Here's how the part is built. I have some questions about the finished solid (model axes, mm). Face numbers are marked on the shaded views. A direction names the side the tool comes from. Give positions to 0.01 mm unless a question says otherwise; leave off trailing zeros. Use one line per item in the form item = value. Start each with the question number.
from build123d import *

# Parameters (mm, degrees)
SKETCH2_R               = 3.127
SKETCH2_W               = 26.7
SKETCH2_H               = 32.3
BOSS_EXTRUDE1_DEPTH     = 10
CUT_EXTRUDE1_DEPTH      = 52.979378239
CUT_EXTRUDE1_DEPTH_BACK = 52.979378239
CUT_EXTRUDE2_DEPTH      = 52.979378239
CUT_EXTRUDE2_DEPTH_BACK = 52.979378239
CUT_EXTRUDE3_REACH      = 60.213
CUT_EXTRUDE3_END_RADIUS = 3.127
SKETCH6_W               = 4.772967813
SKETCH6_H               = 4
CUT_EXTRUDE4_REACH      = 60.213
CUT_EXTRUDE4_END_RADIUS = 3.127
SKETCH7_W               = 4.772967813
SKETCH7_H               = 4
CUT_EXTRUDE5_REACH      = 60.213
CUT_EXTRUDE5_END_RADIUS = 3.127
SKETCH8_W               = 4.772967813
SKETCH8_H               = 4
CUT_EXTRUDE6_REACH      = 60.213
CUT_EXTRUDE6_END_RADIUS = 3.127
SKETCH9_W               = 4.772967813
SKETCH9_H               = 4
SKETCH10_W              = 1.2
SKETCH10_H              = 12.610624374
SKETCH10_W_2            = 7.1
SKETCH10_H_2            = 1.2
SKETCH10_H_3            = 12.7
BOSS_EXTRUDE2_DEPTH     = 4
CUT_EXTRUDE7_DEPTH      = 3
CUT_EXTRUDE9_DEPTH      = 3
SKETCH13_W              = 7.833075365
SKETCH13_H              = 0.6
BOSS_EXTRUDE3_DEPTH     = 1.2
CHAMFER1_SIZE           = 1.2
SKETCH14_W              = 7.833075365
SKETCH14_H              = 0.6
BOSS_EXTRUDE4_DEPTH     = 1.2
CHAMFER2_SIZE           = 1.2


with BuildPart() as part:
    # Sketch2 → Boss-Extrude1 (new body)
    with BuildSketch(Plane(origin=(0, 0, 0), x_dir=(1, 0, 0), z_dir=(0, 1, 0))):
        with BuildLine():
            Line((-34.405486348, 30.435899661), (-24.03957695, 12.074655042))
            Line((-24.03957695, 12.074655042), (-24.03957695, -0.625344958))
            Line((-24.03957695, -0.625344958), (-34.405486348, -18.986589577))
            ThreePointArc((-34.405486348, -18.986589577), (-33.424886075, -24.740002888), (-27.671446386, -23.75955739))
            Line((-27.671446386, -23.75955739), (-13.03957695, -11.625344958))
            Line((-13.03957695, -11.625344958), (-5.93957695, -11.625344958))
            Line((-5.93957695, -11.625344958), (8.692292487, -23.75955739))
            ThreePointArc((8.692292487, -23.75955739), (14.445732176, -24.740002888), (15.426332449, -18.986589577))
            Line((15.426332449, -18.986589577), (5.06042305, -0.625344958))
            Line((5.06042305, -0.625344958), (5.06042305, 12.074655042))
            Line((5.06042305, 12.074655042), (15.426332449, 30.435899661))
            ThreePointArc((15.426332449, 30.435899661), (14.445732176, 36.189312973), (8.692292487, 35.208867474))
            Line((8.692292487, 35.208867474), (-5.93957695, 23.074655042))
            Line((-5.93957695, 23.074655042), (-13.03957695, 23.074655042))
            Line((-13.03957695, 23.074655042), (-27.671446386, 35.208867474))
            ThreePointArc((-27.671446386, 35.208867474), (-33.424886075, 36.189312973), (-34.405486348, 30.435899661))
        make_face()
        with Locations(Location((-31.038402168, 32.82229299, 0), (0, 0, 270))):
            Circle(SKETCH2_R, mode=Mode.SUBTRACT)
        with Locations(Location((12.059248268, 32.82229299, 0), (0, 0, 90))):
            Circle(SKETCH2_R, mode=Mode.SUBTRACT)
        with Locations(Location((-31.038402168, -21.372982906, 0), (0, 0, 90))):
            Circle(SKETCH2_R, mode=Mode.SUBTRACT)
        with Locations(Location((12.059248268, -21.372982906, 0), (0, 0, 270))):
            Circle(SKETCH2_R, mode=Mode.SUBTRACT)
        with BuildLine():
            Line((-24.03957695, 23.074655042), (-14.606114632, 23.074655042))
            Line((-14.606114632, 23.074655042), (-26.939458612, 33.302699824))
            ThreePointArc((-26.939458612, 33.302699824), (-28.459986314, 29.599886951), (-32.406136372, 28.928524617))
            Line((-32.406136372, 28.928524617), (-24.03957695, 14.108749692))
            Line((-24.03957695, 14.108749692), (-24.03957695, 23.074655042))
        make_face(mode=Mode.SUBTRACT)
        with Locations((-9.48957695, 5.724655042)):
            Rectangle(SKETCH2_W, SKETCH2_H, mode=Mode.SUBTRACT)
        with BuildLine():
            Line((5.06042305, 23.074655042), (5.06042305, 14.108749692))
            Line((5.06042305, 14.108749692), (13.426982473, 28.928524617))
            ThreePointArc((13.426982473, 28.928524617), (9.480832414, 29.599886951), (7.960304713, 33.302699824))
            Line((7.960304713, 33.302699824), (-4.373039267, 23.074655042))
            Line((-4.373039267, 23.074655042), (5.06042305, 23.074655042))
        make_face(mode=Mode.SUBTRACT)
        with BuildLine():
            Line((-24.03957695, -11.625344958), (-14.606114632, -11.625344958))
            Line((-14.606114632, -11.625344958), (-26.939458612, -21.85338974))
            ThreePointArc((-26.939458612, -21.85338974), (-28.459986314, -18.150576866), (-32.406136372, -17.479214533))
            Line((-32.406136372, -17.479214533), (-24.03957695, -2.659439608))
            Line((-24.03957695, -2.659439608), (-24.03957695, -11.625344958))
        make_face(mode=Mode.SUBTRACT)
        with BuildLine():
            Line((7.960304713, -21.85338974), (-4.373039267, -11.625344958))
            Line((-4.373039267, -11.625344958), (5.06042305, -11.625344958))
            Line((5.06042305, -11.625344958), (5.06042305, -2.659439608))
            Line((5.06042305, -2.659439608), (13.426982473, -17.479214533))
            ThreePointArc((13.426982473, -17.479214533), (9.480832414, -18.150576866), (7.960304713, -21.85338974))
        make_face(mode=Mode.SUBTRACT)
    extrude(amount=BOSS_EXTRUDE1_DEPTH)

    # Sketch4 → Cut-Extrude1 (cut, two sides: drawn at the far end of the back side and taken through both)
    with BuildSketch(Plane(origin=(0, 0, 0), x_dir=(0, 0, -1), z_dir=(1, 0, 0)).offset(-CUT_EXTRUDE1_DEPTH_BACK)):
        Polygon((-18.986589577, 5), (-18.986589577, 7), (30.435899661, 7), (30.435899661, 5), (30.435899661, 3), (-18.986589577, 3), align=None)
    extrude(amount=CUT_EXTRUDE1_DEPTH + CUT_EXTRUDE1_DEPTH_BACK, mode=Mode.SUBTRACT)

    # Sketch5 → Cut-Extrude2 (cut, two sides: drawn at the far end of the back side and taken through both)
    with BuildSketch(Plane.XY.offset(-CUT_EXTRUDE2_DEPTH_BACK)):
        Polygon((-27.671446386, 5), (-27.671446386, 7), (8.692292487, 7), (8.692292487, 5), (8.692292487, 3), (-27.671446386, 3), align=None)
    extrude(amount=CUT_EXTRUDE2_DEPTH + CUT_EXTRUDE2_DEPTH_BACK, mode=Mode.SUBTRACT)

    # Cut-Extrude3: up to this cylinder (the profile starts outside it)
    cut_extrude3_end = Plane(origin=(-31.038402168, 5, -32.82229299), z_dir=(0, -1, 0)) * Cylinder(CUT_EXTRUDE3_END_RADIUS, 127.68, mode=Mode.PRIVATE)
    # Sketch6 → Cut-Extrude3 (cut, up to the surface)
    with BuildSketch(Plane(origin=(-27.671446386, 0, 0), x_dir=(0, 0, -1), z_dir=(1, 0, 0)), mode=Mode.PRIVATE) as cut_extrude3_sk1:
        with Locations((32.822383567, 5)):
            Rectangle(SKETCH6_W, SKETCH6_H)
    cut_extrude3_tool1 = extrude(cut_extrude3_sk1.sketch, amount=-CUT_EXTRUDE3_REACH, mode=Mode.PRIVATE) - cut_extrude3_end
    add(cut_extrude3_tool1.solids().sort_by_distance((-27.671446, 5, -32.822384))[0], mode=Mode.SUBTRACT)

    # Cut-Extrude4: up to this cylinder (the profile starts outside it)
    cut_extrude4_end = Plane(origin=(-31.038402168, 5, 21.372982906), z_dir=(0, -1, 0)) * Cylinder(CUT_EXTRUDE4_END_RADIUS, 127.68, mode=Mode.PRIVATE)
    # Sketch7 → Cut-Extrude4 (cut, up to the surface)
    with BuildSketch(Plane(origin=(-27.671446386, 0, 0), x_dir=(0, 0, -1), z_dir=(1, 0, 0)), mode=Mode.PRIVATE) as cut_extrude4_sk1:
        with Locations((-21.373073484, 5)):
            Rectangle(SKETCH7_W, SKETCH7_H)
    cut_extrude4_tool1 = extrude(cut_extrude4_sk1.sketch, amount=-CUT_EXTRUDE4_REACH, mode=Mode.PRIVATE) - cut_extrude4_end
    add(cut_extrude4_tool1.solids().sort_by_distance((-27.671446, 5, 21.373073))[0], mode=Mode.SUBTRACT)

    # Cut-Extrude5: up to this cylinder (the profile starts outside it)
    cut_extrude5_end = Plane(origin=(12.059248268, 5, -32.82229299), z_dir=(0, -1, 0)) * Cylinder(CUT_EXTRUDE5_END_RADIUS, 127.68, mode=Mode.PRIVATE)
    # Sketch8 → Cut-Extrude5 (cut, up to the surface)
    with BuildSketch(Plane.ZY.offset(-8.692292487), mode=Mode.PRIVATE) as cut_extrude5_sk1:
        with Locations((-32.822383567, 5)):
            Rectangle(SKETCH8_W, SKETCH8_H)
    cut_extrude5_tool1 = extrude(cut_extrude5_sk1.sketch, amount=-CUT_EXTRUDE5_REACH, mode=Mode.PRIVATE) - cut_extrude5_end
    add(cut_extrude5_tool1.solids().sort_by_distance((8.692292, 5, -32.822384))[0], mode=Mode.SUBTRACT)

    # Cut-Extrude6: up to this cylinder (the profile starts outside it)
    cut_extrude6_end = Plane(origin=(12.059248268, 5, 21.372982906), z_dir=(0, -1, 0)) * Cylinder(CUT_EXTRUDE6_END_RADIUS, 127.68, mode=Mode.PRIVATE)
    # Sketch9 → Cut-Extrude6 (cut, up to the surface)
    with BuildSketch(Plane.ZY.offset(-8.692292487), mode=Mode.PRIVATE) as cut_extrude6_sk1:
        with Locations((21.373073484, 5)):
            Rectangle(SKETCH9_W, SKETCH9_H)
    cut_extrude6_tool1 = extrude(cut_extrude6_sk1.sketch, amount=-CUT_EXTRUDE6_REACH, mode=Mode.PRIVATE) - cut_extrude6_end
    add(cut_extrude6_tool1.solids().sort_by_distance((8.692292, 5, 21.373073))[0], mode=Mode.SUBTRACT)

    # Sketch10 → Boss-Extrude2 (add)
    with BuildSketch(Plane(origin=(0, 3, 0), x_dir=(1, 0, 0), z_dir=(0, 1, 0))):
        with Locations((-23.43957695, 5.769342855)):
            Rectangle(SKETCH10_W, SKETCH10_H)
        with Locations((-9.48957695, 22.474655042)):
            Rectangle(SKETCH10_W_2, SKETCH10_H_2)
        with Locations((4.46042305, 5.724655042)):
            Rectangle(SKETCH10_W, SKETCH10_H_3)
        with Locations((-9.48957695, -11.025344958)):
            Rectangle(SKETCH10_W_2, SKETCH10_H_2)
    extrude(amount=BOSS_EXTRUDE2_DEPTH)

    # Sketch11 → Cut-Extrude7 (cut)
    with BuildSketch(Plane.XZ):
        with BuildLine():
            ThreePointArc((9.773467047, -30.688438916), (10.235471064, -30.282221002), (10.768064045, -29.974316112))
            Line((10.768064045, -29.974316112), (10.176165075, -29.14994678))
            ThreePointArc((10.176165075, -29.14994678), (9.652235629, -29.469917839), (9.181568077, -29.864069585))
            Line((9.181568077, -29.864069585), (9.773467047, -30.688438916))
        make_face()
        with BuildLine():
            ThreePointArc((-28.160721976, -29.864069585), (-28.631389528, -29.469917839), (-29.155318974, -29.14994678))
            Line((-29.155318974, -29.14994678), (-29.747217945, -29.974316112))
            ThreePointArc((-29.747217945, -29.974316112), (-29.214624963, -30.282221002), (-28.752620946, -30.688438916))
            Line((-28.752620946, -30.688438916), (-28.160721976, -29.864069585))
        make_face()
        with BuildLine():
            Line((-28.160721976, 18.414759501), (-28.752620946, 19.239128832))
            ThreePointArc((-28.752620946, 19.239128832), (-29.214624963, 18.832910917), (-29.747217945, 18.525006027))
            Line((-29.747217945, 18.525006027), (-29.155318974, 17.700636696))
            ThreePointArc((-29.155318974, 17.700636696), (-28.631389528, 18.020607755), (-28.160721976, 18.414759501))
        make_face()
        Polygon((11.073162581, 18.949933064), (9.804267287, 17.182674769), (8.809670289, 17.896797574), (10.078565582, 19.664055869), align=None)
    extrude(amount=-CUT_EXTRUDE7_DEPTH, mode=Mode.SUBTRACT)

    # Sketch12 → Cut-Extrude9 (cut)
    with BuildSketch(Plane(origin=(0, 10, 0), x_dir=(1, 0, 0), z_dir=(0, 1, 0))):
        Polygon((-14.606114632, 23.074655042), (-13.406114632, 21.874655042), (-15.406114632, 21.874655042), (-16.606114632, 23.074655042), align=None)
        Polygon((-3.573039267, 21.874655042), (-2.373039267, 23.074655042), (-4.373039267, 23.074655042), (-5.573039267, 21.874655042), align=None)
        Polygon((-15.406114632, -10.425344958), (-16.606114632, -11.625344958), (-14.606114632, -11.625344958), (-13.406114632, -10.425344958), align=None)
        Polygon((-5.573039267, -10.425344958), (-3.573039267, -10.425344958), (-2.373039267, -11.625344958), (-4.373039267, -11.625344958), align=None)
    extrude(amount=-CUT_EXTRUDE9_DEPTH, mode=Mode.SUBTRACT)

    # Sketch13 → Boss-Extrude3 (add)
    with BuildSketch(Plane.XY.offset(-21.874655042)):
        with Locations((-9.48957695, 7.3)):
            Rectangle(SKETCH13_W, SKETCH13_H)
    extrude(amount=BOSS_EXTRUDE3_DEPTH)

    # Chamfer1
    chamfer1_edges = [part.edges().sort_by_distance(p)[0] for p in [
        (-9.48957695, 7, -21.874655042),
    ]]
    chamfer(chamfer1_edges, length=CHAMFER1_SIZE - 0.0001)  # a hair under: the kernel refuses the full size

    # Sketch14 → Boss-Extrude4 (add)
    with BuildSketch(Plane(origin=(0, 0, 10.425344958), x_dir=(-1, 0, 0), z_dir=(0, 0, -1))):
        with Locations((9.48957695, 7.3)):
            Rectangle(SKETCH14_W, SKETCH14_H)
    extrude(amount=BOSS_EXTRUDE4_DEPTH)

    # Chamfer2
    chamfer2_edges = [part.edges().sort_by_distance(p)[0] for p in [
        (-9.48957695, 7, 10.425344958),
    ]]
    chamfer(chamfer2_edges, length=CHAMFER2_SIZE - 0.0001)  # a hair under: the kernel refuses the full size


solid = part.part
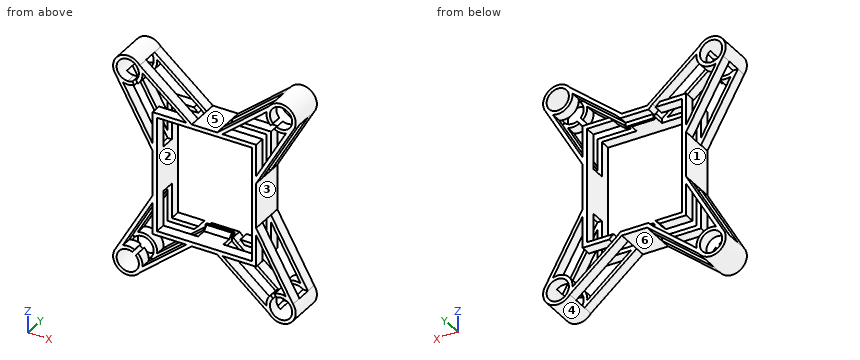
1) On a 3-axis mill with a long thin cutter (end or side, diameter ignored), from which of +Z, -Z, +X, -X, +Y, -Y can I reach the whole of each face in a straight line? I mean the marked faces 1, 2 and 3. Say none if no direction works.
2) Please list where these lines run through material, in increasing order: line 1 (X direction, y = 9.5, z = -11); line 2 (X direction, y = 1.25, z = 9); line 3 (Y direction, x = -2, z = -25.5).
3) Thinking about a two-plate mould opening in Z: for the marked faces 4, 5 and 6, which applies, released by +Z, released by -Z, zero draft, split by the parting line, or undercut?
4) Will these pins go through, and if not, where does the flat tip stop? P1, Ø6, axis at y = 6.5, z = -16, coming from the +X side; P2, Ø1.5, axis at x = -0.5, y = 8.5, coming from the -Z side; P3, Ø1.5, axis at y = 1.5, z = -20, coming from the +X side.
5) Suppose I cut it at A-A, the plane y = 5. State how many separate pieces and enclosed holes the cut face has, and give its area (3 significant figures).
Checks:
q1.face_1 = -X, +Y, -Y
q1.face_2 = +Y, -Y
q1.face_3 = +X, +Y, -Y
q2.line_1 = -24.04 to -22.84, 3.86 to 5.06
q2.line_2 = -28.77 to -27.62, -24.04 to -22.84, 3.86 to 5.06, 8.64 to 9.79
q2.line_3 = 0 to 3, 7 to 10
q3.face_4 = undercut
q3.face_5 = released by +Z
q3.face_6 = released by -Z
q4.P1 = 8.95
q4.P2 = -28.21
q4.P3 = 9.96
q5.separate_pieces = 8
q5.enclosed_holes = 0
q5.area = 93.0 mm^2
